Verification items for the finished model (mm, model axes). A direction names the side the tool comes from. Give positions to 0.01 mm unless a question says otherwise; leave off trailing zeros. Write each loop counter-clockwise with the first axis right and the second up, starting at its lowest first coordinate (ties: lowest second). Pieces come first, ordered by that corner, then holes. Notation, with made-up numbers: M 28.5,50.5 L 39.5,50.5 A37 cw 39.5,88.5 Z; hole C -7,43.25 d9. An arc over 180 degrees is marked long. Answer as a JSON object with one key per item and string values.
```python
from build123d import *

# Parameters (mm, degrees)
F0_R     = 11
F0_R_2   = 4
F1_DEPTH = 5
F2_DEPTH = 10
F3_SIZE  = 0.8


with BuildPart() as f1:
    # F0 (on Top) → F1 (new body)
    with BuildSketch(Plane.XY):
        with BuildLine():
            Line((-1.3099432081, 16), (-6, 16))
            ThreePointArc((-6, 16), (-13.0710678119, 13.0710678119), (-16, 6))
            Line((-16, 6), (-16, -6))
            ThreePointArc((-16, -6), (-13.0710678119, -13.0710678119), (-6, -16))
            Line((-6, -16), (-1.3099432081, -16))
            ThreePointArc((-1.3099432081, -16), (-0.0172155068, -15.8948625758), (1.2415336792, -15.5822137726))
            Line((1.2415336792, -15.5822137726), (23.5514768872, -8.074735593))
            ThreePointArc((23.5514768872, -8.074735593), (27.4966073876, -5.1609361605), (29, -0.4925218204))
            Line((29, -0.4925218204), (29, 0.4925218204))
            ThreePointArc((29, 0.4925218204), (27.4966073876, 5.1609361605), (23.5514768872, 8.074735593))
            Line((23.5514768872, 8.074735593), (1.2415336792, 15.5822137726))
            ThreePointArc((1.2415336792, 15.5822137726), (-0.0172155068, 15.8948625758), (-1.3099432081, 16))
        make_face()
        Circle(F0_R, mode=Mode.SUBTRACT)
        with Locations((20, 0)):
            Circle(F0_R_2, mode=Mode.SUBTRACT)
        with Locations((20, 0)):
            Circle(F0_R_2)
    extrude(amount=F1_DEPTH)

    # F0 (on Top) → F2 (join, through all)
    with BuildSketch(Plane.XY):
        with Locations((20, 0)):
            Circle(F0_R_2)
    extrude(amount=F2_DEPTH)

    # F3
    f3_edges = [f1.edges().sort_by_distance(p)[0] for p in [
        (16, 0, 10),
        (-11, 0, 5),
    ]]
    chamfer(f3_edges, length=F3_SIZE)


solid = f1.part
```
1) Go/stop test with flat-tipped pins: pin 1 (6 mm diameter, centred on x = -3.5, y = 6, fed in from +Z); pin 2 (2 mm diameter, centred on y = 11.5, z = 5.5, fed in from -X); pin 3 (4 mm diameter, centred on x = 16, z = 8, fed in from +Y); pin 4 (1 mm diameter, centred on x = 5, z = 3, fed in from -Y). Record where each tip stops, or that it passes through.
Completed:
{"pin 1": "passes through", "pin 2": "stops at x = -14.86", "pin 3": "stops at y = 3.46", "pin 4": "stops at y = -14.49"}
2) Thickness scan on L1, parallel to Z at x = 15.5, y = 2.5; L2, parallel to Y at x = -2.5, z = 4.25; L3, parallel to Y at x = 0, z = 2.65. Record the ranges inside material, lowest first.
Completed:
{"L1": "z = 0 to 5", "L2": "y = -16 to -10.76, 10.76 to 16", "L3": "y = -15.89 to -11, 11 to 15.89"}
3) Release check for a two-part mould opening along Y. For faces 3 (the face through (-0.04, -15.9, 2.46)), 4 (the face through (-12.99, 13.15, 2.46)), 5 (the face through (-2.38, -10.74, 2.07)) record: pulls with the +Y half, pulls with the -Y half, needs draft (parallel to the pull), parting line crosses it, or undercut.
Completed:
{"face 3": "pulls with the -Y half", "face 4": "pulls with the +Y half", "face 5": "undercut"}
4) Section check C-C on x = 0. Record the boundary of the cut face in (y, z), and give its area (3 significant figures).
Completed:
{"outline": "M -15.89,0 L -11,0 L -11,4.2 L -11.8,5 L -15.89,5 Z; M 11,0 L 15.89,0 L 15.89,5 L 11.8,5 L 11,4.2 Z", "area": "48.3 mm2"}
5) Section check D-D on x = 20. Record the boundary of the cut face in (y, z).
Completed:
{"outline": "M -9.27,0 L 9.27,0 L 9.27,5 L 4,5 L 4,9.2 L 3.2,10 L -3.2,10 L -4,9.2 L -4,5 L -9.27,5 Z"}
6) Access from +Z, -Z, +X, -X, +Y, -Y to the whole of each face (thin tool, end or side, straight path). Record for faces 1 (the face through (16.8, -2.4, 7.1)), 2 (the face through (12.24, -11.88, 2.46)).
Completed:
{"face 1": "+Z", "face 2": "+Z, -Z, +X, -Y"}
7) Section check B-B on z = 3.25. Record the boundary of the cut face in (x, y).
Completed:
{"outline": "M -16,-6 A10 ccw -6,-16 L -1.31,-16 A8 ccw 1.24,-15.58 L 23.55,-8.07 A8 ccw 29,-0.49 L 29,0.49 A8 ccw 23.55,8.07 L 1.24,15.58 A8 ccw -1.31,16 L -6,16 A10 ccw -16,6 Z; hole C 0,0 d22"}
8) Section check A-A on y = 0. Record the boundary of the cut face in (x, z), and give its area (3 significant figures).
Completed:
{"outline": "M -16,0 L -11,0 L -11,4.2 L -11.8,5 L -16,5 Z; M 11,0 L 29,0 L 29,5 L 24,5 L 24,9.2 L 23.2,10 L 16.8,10 L 16,9.2 L 16,5 L 11.8,5 L 11,4.2 Z", "area": "154 mm2"}
